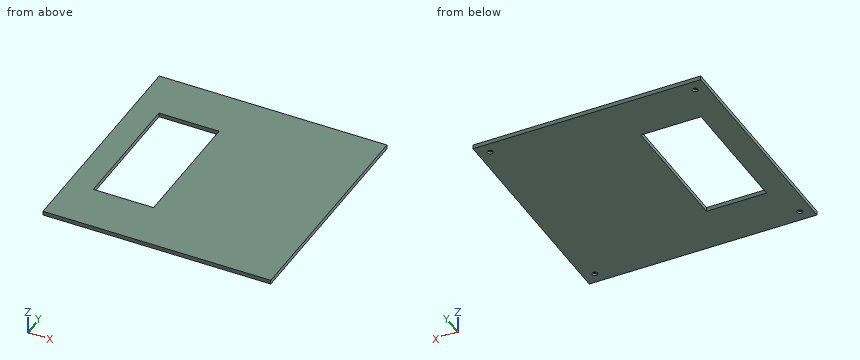
from build123d import *

# Parameters (mm, degrees)
F0_W     = 500
F0_H     = 500
F0_R     = 6
F0_W_2   = 132
F0_H_2   = 282
F0_R_2   = 3.1
F1_DEPTH = 9
F2_DEPTH = 7
F3_DEPTH = 5
F4_DEPTH = 25


with BuildPart() as f1:
    # F0 (on Top) → F1 (new body)
    with BuildSketch(Plane.XY):
        with Locations((250, 250)):
            Rectangle(F0_W, F0_H)
        with Locations((25, 25)):
            Circle(F0_R, mode=Mode.SUBTRACT)
        with Locations((475, 25)):
            Circle(F0_R, mode=Mode.SUBTRACT)
        with Locations((121, 250)):
            Rectangle(F0_W_2, F0_H_2, mode=Mode.SUBTRACT)
        with Locations((25, 475)):
            Circle(F0_R, mode=Mode.SUBTRACT)
        with Locations((475, 475)):
            Circle(F0_R, mode=Mode.SUBTRACT)
        with Locations((121, 250)):
            Rectangle(F0_W_2, F0_H_2)
        with Locations((475, 25)):
            Circle(F0_R)
        with Locations((475, 25)):
            Circle(F0_R_2, mode=Mode.SUBTRACT)
        with Locations((25, 25)):
            Circle(F0_R)
        with Locations((25, 25)):
            Circle(F0_R_2, mode=Mode.SUBTRACT)
        with Locations((25, 475)):
            Circle(F0_R)
        with Locations((25, 475)):
            Circle(F0_R_2, mode=Mode.SUBTRACT)
        with Locations((475, 475)):
            Circle(F0_R)
        with Locations((475, 475)):
            Circle(F0_R_2, mode=Mode.SUBTRACT)
        with Locations((475, 25)):
            Circle(F0_R_2)
        with Locations((475, 475)):
            Circle(F0_R_2)
        with Locations((25, 475)):
            Circle(F0_R_2)
        with Locations((25, 25)):
            Circle(F0_R_2)
    extrude(amount=F1_DEPTH)

    # F0 (on Top) → F2 (cut)
    with BuildSketch(Plane.XY):
        with Locations((475, 25)):
            Circle(F0_R_2)
        with Locations((475, 475)):
            Circle(F0_R_2)
        with Locations((25, 475)):
            Circle(F0_R_2)
        with Locations((25, 25)):
            Circle(F0_R_2)
    extrude(amount=F2_DEPTH, mode=Mode.SUBTRACT)

    # F0 (on Top) → F3 (cut)
    with BuildSketch(Plane.XY):
        with Locations((475, 475)):
            Circle(F0_R)
        with Locations((475, 475)):
            Circle(F0_R_2, mode=Mode.SUBTRACT)
        with Locations((25, 475)):
            Circle(F0_R)
        with Locations((25, 475)):
            Circle(F0_R_2, mode=Mode.SUBTRACT)
        with Locations((25, 25)):
            Circle(F0_R)
        with Locations((25, 25)):
            Circle(F0_R_2, mode=Mode.SUBTRACT)
        with Locations((475, 25)):
            Circle(F0_R)
        with Locations((475, 25)):
            Circle(F0_R_2, mode=Mode.SUBTRACT)
    extrude(amount=F3_DEPTH, mode=Mode.SUBTRACT)

    # F0 (on Top) → F4 (cut)
    with BuildSketch(Plane.XY):
        with Locations((121, 250)):
            Rectangle(F0_W_2, F0_H_2)
    extrude(amount=F4_DEPTH, mode=Mode.SUBTRACT)


solid = f1.part
Input: part model. Units: mm. Frame: model coordinates. Give positions to 0.01 mm unless a question says otherwise; leave off trailing zeros. Loops run counter-clockwise (first coordinate to the right, second up) from the corner with the lowest first, then second, coordinate; pieces in that order, holes last. Notation, with made-up numbers: M 80.25,48 L 110.25,48 A16 ccw 110.25,68 Z; hole C 30.5,84 d11. An arc over 180 degrees is marked long. Use CSV: the item, a comma, the result in double quotes.
(1) Material intervals for L1, parallel to Y at x = 475, z = 6.5; L2, parallel to Y at x = 25, z = 3.85, sorted ascending. Write a range as [from, to].
Outcome:
L1,"y = [0, 21.9], [28.1, 471.9], [478.1, 500]"
L2,"y = [0, 19], [31, 469], [481, 500]"
(2) Section A-A, the plane x = 122.5. Return loops of the section in (y, z).
Outcome:
outline,"M 0,0 L 109,0 L 109,9 L 0,9 Z; M 391,0 L 500,0 L 500,9 L 391,9 Z"
(3) Section B-B, the plane y = 345. Return loops of the section in (x, z), plus the area to 3 significant figures.
Outcome:
outline,"M 0,0 L 55,0 L 55,9 L 0,9 Z; M 187,0 L 500,0 L 500,9 L 187,9 Z"
area,"3,310 mm²"
(4) Pin query (flat end, axial travel): P1, Ø5.5, axis at x = 25, y = 25, coming from the -Z side; P2, Ø9.5, axis at x = 475.5, y = 476, coming from the -Z side. Return the tip coordinate at first contact, or that it passes through.
Outcome:
P1,"stops at z = 7"
P2,"stops at z = 5"
